Geometry check sheet. Reference: the model listing, model coordinates, mm. A direction names the side the tool comes from. Round coordinates to 2 decimals unless told otherwise and drop trailing zeros. Loops run counter-clockwise (first coordinate to the right, second up) from the corner with the lowest first, then second, coordinate; pieces in that order, holes last. Notation, with made-up numbers: (77, -27.5) -> (88, -27.5) arc R11 cw to (88, -21.5) -> close; hole circle Ø9 at (51.25, 11.5). An arc over 180 degrees is marked (long way). Use a Markdown table: item, result. Add a question column.
Q1. Material ranges on L1, parallel to Z at x = 0.5, y = 0.8; L2, parallel to X at y = 1.5, z = 2.5, recorded low to high.
Q2. Gauge pin test, flat ends, axial feed: P1, Ø0.8, axis at y = 2, z = 1, coming from the -X side; P2, Ø1.4, axis at y = 2, z = 0.5, coming from the +X side; P3, Ø1, axis at x = 0, y = 2, coming from the +Z side. Record the tip position at first contact, or that the pin passes through.
Q3. Release check for a two-part mould opening along X. For faces 6 (the face through (0, 2, -4.1)), 7 (the face through (0, 3.2, 0)), 8 (the face through (-4.8, 0.5, -0.1)) record: released by +X, released by -X, zero draft, split by the parting line, or undercut.
Q4. Sectioned sample at C-C, the plane z = 1.25. Enter the section's corners in (x, y), then the cut area to 3 significant figures.
Q5. Sectioned sample at B-B, the plane x = -2.5. Enter the section's corners in (y, z), then the cut area to 3 significant figures.
Q6. Set-up check for faces 1 (the face through (-4.1, 2, 0)), 2 (the face through (0, 2, 4.1)), 3 (the face through (-3.3, 2, 0)), 4 (the face through (0, 5, 0)), 5 (the face through (-0.057, 4.715, -3.799)): record each of +Z, -Z, +X, -X, +Y, -Y from which the full face is reachable in a straight line by a thin tool's end or side.
Q7. Sectioned sample at A-A, the plane y = 2.7. Enter the section's corners in (x, z), then the cut area to 3 significant figures.
Q8. Sectioned sample at D-D, the plane y = 3.7. Enter the section's corners in (x, z).
Autodesk Inventor part; units mm, degrees
ref_plane "YZ Plane" through (0, 0, 0) normal (1, 0, 0) x (0, 1, 0)
ref_plane "XZ Plane" through (0, 0, 0) normal (0, 1, 0) x (-1, 0, 0)
ref_plane "XY Plane" through (0, 0, 0) normal (0, 0, 1) x (1, 0, 0)
sketch "Эскиз1" plane through (0, 0, 0) normal (0, 1, 0) x (-1, 0, 0)
  line L0 (4.1, 4.1) -> (-4.1, 4.1)
  line L1 (-4.1, 4.1) -> (-4.1, -4.1)
  line L2 (-4.1, -4.1) -> (4.1, -4.1)
  line L3 (4.1, -4.1) -> (4.1, 4.1)
  line L4 (5.74, 0) -> (-5.74, 0)
  line L5 (0, -5.74) -> (0, 5.74)
  point P0 (0, 0)
  dimension "d0" = 8.2
extrude "Выдавливание1" add sketch "Эскиз1" along normal blind 5
shell "Оболочка1" thickness 0.8 removed faces 1 at (1.3667, 0, 1.3667)
sketch "Эскиз3" plane through (-3.3, 4.2, 3.3) normal (0, -1, 0) x (1, 0, 0)
  line L0 (0, 0) -> (6.6, 0)
  line L1 (6.6, -6.6) -> (0, -6.6)
  line L2 (6.6, 0) -> (0, 0)
  line L3 (0, 0) -> (0, -6.6)
  line L4 (0, -6.6) -> (6.6, -6.6)
  line L5 (6.6, -6.6) -> (6.6, 0)
  point P0 (3.3, -3.3)
extrude "Выдавливание2" add sketch "Эскиз3" along normal blind 1
fillet "Сопряжение1" radius 1 4 edges at (0, 5, -4.1) (0, 5, 4.1) (4.1, 5, 0) (-4.1, 5, 0)
sketch "Эскиз5" plane through (0, 0, 0) normal (0, -1, 0) x (1, 0, 0)
  line L0 (-4.1, 4.1) -> (4.1, 4.1)
  line L1 (4.1, 4.1) -> (4.1, -4.1)
  line L2 (4.1, -4.1) -> (-4.1, -4.1)
  line L3 (-4.1, -4.1) -> (-4.1, 4.1)
  line L4 (-4.6, -4.6) -> (4.6, -4.6)
  line L5 (4.6, -4.6) -> (4.6, 4.6)
  line L6 (4.6, 4.6) -> (-4.6, 4.6)
  line L7 (-4.6, 4.6) -> (-4.6, -4.6)
  line L8 (4.6, -4.6) -> (4.8, -4.6)
  line L9 (4.8, -4.6) -> (4.8, 4.6)
  line L10 (4.8, 4.6) -> (4.6, 4.6)
  line L11 (4.6, 4.6) -> (4.6, -4.6)
  line L12 (-4.6, -4.6) -> (-4.8, -4.6)
  line L13 (-4.8, -4.6) -> (-4.8, 4.6)
  line L14 (-4.8, 4.6) -> (-4.6, 4.6)
  line L15 (-4.6, 4.6) -> (-4.6, -4.6)
  point P0 (0, 0)
  dimension "d10" = 0.5
  dimension "d13" = 0.2
  dimension "d14" = 0.2
extrude "Выдавливание4" add sketch "Эскиз5" against normal blind 1
chamfer "Фаска1" distance 0.5 angle 45 4 edges at (-3.3, 0, 0) (0, 0, 3.3) (3.3, 0, 0) (0, 0, -3.3)
properties part number "BUTTON2"
Values:
| question | item | result |
|---|---|---|
| 1 | L1 | -4.6 to -3.3, 3.3 to 4.6 |
| 1 | L2 | -4.1 to -3.3, 3.3 to 4.1 |
| 2 | P1 | x = -4.1 |
| 2 | P2 | x = 4.1 |
| 2 | P3 | z = 4.1 |
| 3 | face 6 | zero draft |
| 3 | face 7 | undercut |
| 3 | face 8 | released by -X |
| 4 | outline | (-4.8, 0) -> (-3.8, 0) -> (-3.3, 0.5) -> (-3.3, 3.2) -> (3.3, 3.2) -> (3.3, 0.5) -> (3.8, 0) -> (4.8, 0) -> (4.8, 1) -> (4.1, 1) -> (4.1, 4) arc R1 ccw to (3.1, 5) -> (-3.1, 5) arc R1 ccw to (-4.1, 4) -> (-4.1, 1) -> (-4.8, 1) -> close |
| 4 | area | 20.6 mm^2 |
| 5 | outline | (0, -4.6) -> (1, -4.6) -> (1, -4.1) -> (4, -4.1) arc R1 ccw to (5, -3.1) -> (5, 3.1) arc R1 ccw to (4, 4.1) -> (1, 4.1) -> (1, 4.6) -> (0, 4.6) -> (0, 3.8) -> (0.5, 3.3) -> (3.2, 3.3) -> (3.2, -3.3) -> (0.5, -3.3) -> (0, -3.8) -> close |
| 5 | area | 20.2 mm^2 |
| 6 | face 1 | +Z, -Z, -X, +Y |
| 6 | face 2 | +Z, +X, -X, +Y |
| 6 | face 3 | -Y |
| 6 | face 4 | +Z, -Z, +X, -X, +Y |
| 6 | face 5 | -Z, +X, -X, +Y |
| 7 | outline | (-4.1, -4.1) -> (4.1, -4.1) -> (4.1, 4.1) -> (-4.1, 4.1) -> close; hole (-3.3, -3.3) -> (3.3, -3.3) -> (3.3, 3.3) -> (-3.3, 3.3) -> close |
| 7 | area | 23.7 mm^2 |
| 8 | outline | (-4.1, -4.1) -> (4.1, -4.1) -> (4.1, 4.1) -> (-4.1, 4.1) -> close |
